Check sheet for the modelled part. Datum: model origin and axes. Units: mm. A direction names the side the tool comes from. Give positions to 0.01 mm unless a question says otherwise; leave off trailing zeros. Order: outer loops, then holes, each group sorted by start corner. A loop starts at its lowest first (then second) coordinate and runs counter-clockwise, first axis right, second up.
Item 1: Sectioned sample at A-A on z = 5. Record the boundary of the cut face in (x, y).
Item 2: Material ranges on line 1 along Y through (x, z) = (47, 21); line 2 along X through (y, z) = (65, 8.25); line 3 along Z through (x, y) = (55.5, 5.5), recorded low to high.
Item 3: Access from +Z, -Z, +X, -X, +Y, -Y to the whole of each face (thin tool, end or side, straight path). Record for faces 5 (the flat face through (38, 66, 14)), 6 (the flat face through (38, 68, 12)).
Item 4: Sectioned sample at B-B on y = 7.5. Record the boundary of the cut face in (x, z).
Item 5: Sectioned sample at C-C on z = 12.75. Record the boundary of the cut face in (x, y), and give its area (3 significant figures).
Item 6: Release check for a two-part mould opening along X. For faces 1 (the cylindrical face through (68.5, 7.5, 5.5)), 2 (the flat face through (77, 33, 12)), 3 (the flat face through (38, -2, 12)), 4 (the flat face through (37, 33, 4)) record: released by +X, released by -X, zero draft, split by the parting line, or undercut.
Item 7: Sectioned sample at D-D on x = 11. Record the boundary of the cut face in (y, z), and give its area (3 significant figures).
Item 8: Gauge pin test, flat ends, axial feed: P1, Ø1.6, axis at x = 68, y = 58, coming from the +Z side; P2, Ø20, axis at x = 47, y = 28.5, coming from the +Z side. Record the tip position at first contact, or that the pin passes through.
from build123d import *

# Parameters (mm, degrees)
ESQUISSE1_W        = 75
ESQUISSE1_H        = 66
BOSS_EXTRU_1_DEPTH = 4
ESQUISSE2_R        = 1
BOSS_EXTRU_2_DEPTH = 3
ESQUISSE3_W        = 79
ESQUISSE3_H        = 70
ESQUISSE3_W_2      = 75
ESQUISSE3_H_2      = 66
BOSS_EXTRU_3_DEPTH = 25


with BuildPart() as part:
    # Esquisse1 → Boss.-Extru.1 (new body)
    with BuildSketch(Plane.XY):
        with Locations((37.5, 33)):
            Rectangle(ESQUISSE1_W, ESQUISSE1_H)
    extrude(amount=BOSS_EXTRU_1_DEPTH)

    # Esquisse2 → Boss.-Extru.2 (add)
    with BuildSketch(Plane.XY.offset(4)):
        with Locations(Location((67.5, 7.5, 0), (0, 0, 180))):
            Circle(ESQUISSE2_R)
        with Locations(Location((67.5, 58.5, 0), (0, 0, 180))):
            Circle(ESQUISSE2_R)
        with Locations(Location((7.5, 58.5, 0), (0, 0, 180))):
            Circle(ESQUISSE2_R)
        with Locations(Location((7.5, 7.5, 0), (0, 0, 180))):
            Circle(ESQUISSE2_R)
    extrude(amount=BOSS_EXTRU_2_DEPTH)

    # Esquisse3 → Boss.-Extru.3 (add)
    with BuildSketch(Plane(origin=(0, 0, 0), x_dir=(-1, 0, 0), z_dir=(0, 0, -1))):
        with Locations((-37.5, 33)):
            Rectangle(ESQUISSE3_W, ESQUISSE3_H)
        with Locations((-37.5, 33)):
            Rectangle(ESQUISSE3_W_2, ESQUISSE3_H_2, mode=Mode.SUBTRACT)
    extrude(amount=-BOSS_EXTRU_3_DEPTH)


solid = part.part
Report:
1. outline: (-2, -2) - (77, -2) - (77, 68) - (-2, 68) - close; circle Ø2 at (7.5, 7.5); circle Ø2 at (7.5, 58.5); circle Ø2 at (67.5, 7.5); circle Ø2 at (67.5, 58.5); hole (0, 0) - (75, 0) - (75, 66) - (0, 66) - close
2. line 1: y = -2 to 0, 66 to 68
2. line 2: x = -2 to 0, 75 to 77
2. line 3: z = 0 to 4
3. face 5: +Z
3. face 6: +Z, -Z, +X, -X, +Y
4. outline: (-2, 0) - (77, 0) - (77, 25) - (75, 25) - (75, 4) - (68.5, 4) - (68.5, 7) - (66.5, 7) - (66.5, 4) - (8.5, 4) - (8.5, 7) - (6.5, 7) - (6.5, 4) - (0, 4) - (0, 25) - (-2, 25) - close
5. outline: (-2, -2) - (77, -2) - (77, 68) - (-2, 68) - close; hole (0, 0) - (75, 0) - (75, 66) - (0, 66) - close
5. area: 580 mm2
6. face 1: undercut
6. face 2: released by +X
6. face 3: zero draft
6. face 4: undercut
7. outline: (-2, 0) - (68, 0) - (68, 25) - (66, 25) - (66, 4) - (0, 4) - (0, 25) - (-2, 25) - close
7. area: 364 mm2
8. P1: stops at z = 7
8. P2: stops at z = 4
